Read the model definition and answer for the solid it produces. Units are mm, in the model's axes. Face numbers are marked on the shaded views. A direction names the side the tool comes from. Give positions to 0.01 mm unless a question says otherwise; leave off trailing zeros. Write each loop counter-clockwise with the first axis right and the second up, starting at its lowest first coordinate (ties: lowest second). Pieces come first, ordered by that corner, then holes. Notation, with made-up numbers: (29.5, -33.75) -> (43.5, -33.75) arc R19 ccw to (43.5, -20.75) -> close; hole circle Ø1 at (-31, -5.75). An arc over 180 degrees is marked (long way). Use a Markdown table: item, result.
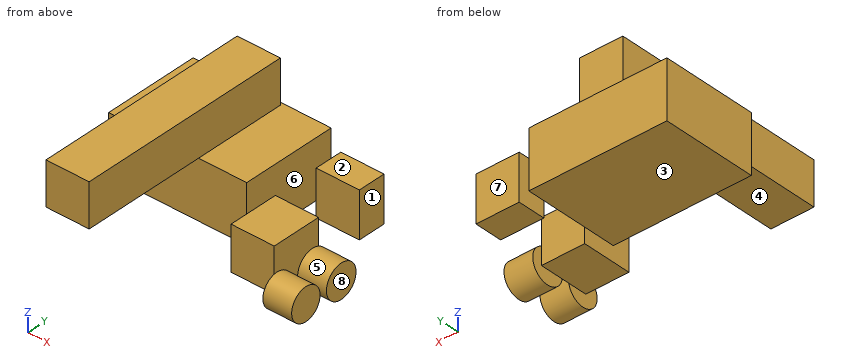
from build123d import *

# Parameters (mm, degrees)
F0_W     = 76.2
F0_H     = 76.2
F1_DEPTH = 381
F4_W     = 243.6232632026
F4_H     = 168.1647449732
F5_DEPTH = 101.6
F6_W     = 88.2032513618
F6_H     = 77.649012208
F6_W_2   = 49.0783378482
F6_H_2   = 80.6645080447
F7_DEPTH = 76.2
F8_R     = 28.3330362408
F8_R_2   = 29.4879309961
F9_DEPTH = 50.8


# Not quite as in the source:
# - the program builds the solid bodies; features that only make, move or delete a surface that nothing else refers to are left out


with BuildPart() as f1:
    # F0 (on Front) → F1 (new body)
    with BuildSketch(Plane.XZ):
        with Locations((-5.1436224073, 48.1359618664)):
            Rectangle(F0_W, F0_H)
    extrude(amount=F1_DEPTH)

    # F4 (on face) → F5 (join)
    with BuildSketch(Plane(origin=(0, 0, 10.0359618664), x_dir=(1, 0, 0), z_dir=(0, 0, -1))):
        with Locations((-3.8859811611, 78.9063498378)):
            Rectangle(F4_W, F4_H)
    extrude(amount=F5_DEPTH)

    # F6 (on face) → F7 (join)
    with BuildSketch(Plane.YZ.offset(117.9256504402)):
        with Locations((-150.0591784716, -79.3707072735)):
            Rectangle(F6_W, F6_H)
        with Locations((0, -79.3707072735)):
            Rectangle(F6_W_2, F6_H_2)
    extrude(amount=F7_DEPTH)

    # F8 (on face) → F9 (join)
    with BuildSketch(Plane.YZ.offset(194.1256504402)):
        with Locations((-188.5067522526, -113.6719733477)):
            Circle(F8_R)
        with Locations((-118.0195510387, -113.6719733477)):
            Circle(F8_R_2)
    extrude(amount=F9_DEPTH)


solid = f1.part
Item 1: A cutting plane is placed at C-C (x = -10). Give the vertices of the cut face in (y, z), then the cut area to 3 significant figures.
Return value:
| item | result |
|---|---|
| outline | (-381, 10.04) -> (-162.99, 10.04) -> (-162.99, -91.56) -> (5.18, -91.56) -> (5.18, 10.04) -> (0, 10.04) -> (0, 86.24) -> (-381, 86.24) -> close |
| area | 46,100 mm^2 |
Item 2: A cutting plane is placed at D-D (z = -48). Give the vertices of the cut face in (x, y), then the cut area to 3 significant figures.
Return value:
| item | result |
|---|---|
| outline | (-125.7, -162.99) -> (117.93, -162.99) -> (117.93, -194.16) -> (194.13, -194.16) -> (194.13, -105.96) -> (117.93, -105.96) -> (117.93, -24.54) -> (194.13, -24.54) -> (194.13, 24.54) -> (117.93, 24.54) -> (117.93, 5.18) -> (-125.7, 5.18) -> close |
| area | 51,400 mm^2 |
Item 3: Each of these flat-tipped pins is pushed along its axis until it touches: P1, Ø6, axis at x = -1.5, y = -138, coming from the -Z side; P2, Ø23, axis at x = 174.5, y = -139, coming from the -Z side; P3, Ø23, axis at x = 138.5, y = -146.5, coming from the +Z side; P4, Ø12, axis at x = 166.5, y = -32.5, coming from the -Z side. Where does it stop, or does it pass through?
Return value:
| item | result |
|---|---|
| P1 | z = -91.56 |
| P2 | z = -118.2 |
| P3 | z = -40.55 |
| P4 | through |
Item 4: A cutting plane is placed at B-B (z = -101.5). Give the vertices of the cut face in (x, y), then the cut area to 3 significant figures.
Return value:
| item | result |
|---|---|
| outline | (117.93, -194.16) -> (194.13, -194.16) -> (194.13, -214.09) -> (244.93, -214.09) -> (244.93, -162.92) -> (194.13, -162.92) -> (194.13, -144.88) -> (244.93, -144.88) -> (244.93, -91.16) -> (194.13, -91.16) -> (194.13, -105.96) -> (117.93, -105.96) -> close; (117.93, -24.54) -> (194.13, -24.54) -> (194.13, 24.54) -> (117.93, 24.54) -> close |
| area | 15,800 mm^2 |
Item 5: For a pull along Y with two mould halves and no side action, classify the marked faces 6, 7 and 8 as +Y half, -Y half, draft (parallel to the pull), parting line (faces both ways), or undercut.
Return value:
| item | result |
|---|---|
| face 6 | undercut |
| face 7 | +Y half |
| face 8 | draft |
Item 6: A tool of negligible diameter and unlimited length cuts with its end or side. For the marked faces 1, 2, 3, 4 and 5, from which of +Z, -Z, +X, -X, +Y, -Y can it reach the whole face along a straight path? Write none if from no direction.
Return value:
| item | result |
|---|---|
| face 1 | +Z, -Z, +X, +Y |
| face 2 | +Z, +X, +Y, -Y |
| face 3 | -Z, -X, +Y, -Y |
| face 4 | -Z, +X, -X, -Y |
| face 5 | +X |
Item 7: Straight lines are drawn through the part: line 1 along X through (y, z) = (-142.5, 63); line 2 along Z through (x, y) = (-22.5, -274); line 3 along Z through (x, y) = (68, -57). For each, find the intervals that lie inside material, in ascending order. Write a range as [from, to].
Return value:
| item | result |
|---|---|
| line 1 | [-43.24, 32.96] |
| line 2 | [10.04, 86.24] |
| line 3 | [-91.56, 10.04] |
Item 8: A cutting plane is placed at A-A (x = 175.5). Give the vertices of the cut face in (y, z).
Return value:
| item | result |
|---|---|
| outline | (-194.16, -118.2) -> (-105.96, -118.2) -> (-105.96, -40.55) -> (-194.16, -40.55) -> close; (-24.54, -119.7) -> (24.54, -119.7) -> (24.54, -39.04) -> (-24.54, -39.04) -> close |
